```python
from build123d import *

# Parameters (mm, degrees)
SKETCH1_R           = 25.4
BOSS_EXTRUDE1_DEPTH = 584.2
SKETCH2_OUTSIDE_W   = 170.52
SKETCH2_OUTSIDE_H   = 170.52
SKETCH2_OUTSIDE_R   = 6.361935525
CUT_EXTRUDE1_DEPTH  = 50.8
SKETCH5_OUTSIDE_W   = 170.52
SKETCH5_OUTSIDE_H   = 170.52
SKETCH5_OUTSIDE_R   = 6.377907631
CUT_EXTRUDE4_DEPTH  = 50.8


with BuildPart() as part:
    # Sketch1 → Boss-Extrude1 (new body)
    with BuildSketch(Plane.XY):
        Circle(SKETCH1_R)
    extrude(amount=BOSS_EXTRUDE1_DEPTH)

    # Sketch2 outside → Cut-Extrude1 (cut)
    with BuildSketch(Plane.XY):
        Rectangle(SKETCH2_OUTSIDE_W, SKETCH2_OUTSIDE_H)
        Circle(SKETCH2_OUTSIDE_R, mode=Mode.SUBTRACT)
    extrude(amount=CUT_EXTRUDE1_DEPTH, mode=Mode.SUBTRACT)

    # Sketch5 outside → Cut-Extrude4 (cut)
    with BuildSketch(Plane.XY.offset(584.2)):
        Rectangle(SKETCH5_OUTSIDE_W, SKETCH5_OUTSIDE_H)
        Circle(SKETCH5_OUTSIDE_R, mode=Mode.SUBTRACT)
    extrude(amount=-CUT_EXTRUDE4_DEPTH, mode=Mode.SUBTRACT)


solid = part.part
```
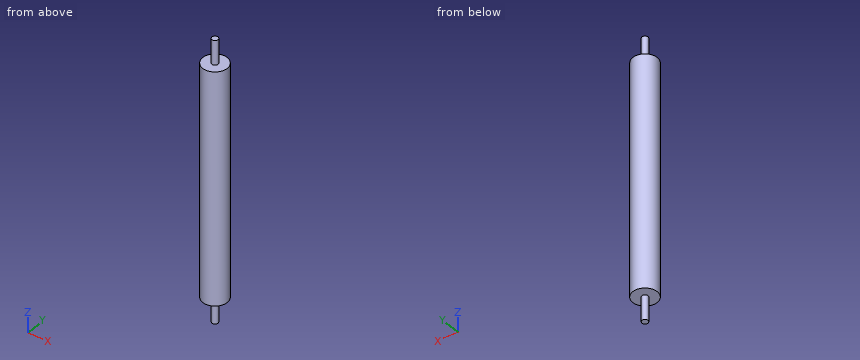
Part model, mm, in its own coordinate system. Round coordinates to 2 decimals unless told otherwise and drop trailing zeros. Order: outer loops, then holes, each group sorted by start corner. A loop starts at its lowest first (then second) coordinate and runs counter-clockwise, first axis right, second up. Notation, with made-up numbers: M -5.5,5.25 L -0.5,5.25 A8 ccw -0.5,17.25 Z; hole C 19,-1 d8. An arc over 180 degrees is marked long. Answer in a Markdown table with one row per item. Add a question column.
Q1. Cut at D-D on z = 539.5. Give the cut face in (x, y), and give its area (3 significant figures).
Q2. Pin check, flat tips, straight feed: pin 1 (10 mm diameter, centred on x = -3, y = -17, fed in from -Z); pin 2 (12 mm diameter, centred on x = 8, y = 11.5, fed in from +Z); pin 3 (10 mm diameter, centred on x = -14.5, z = 146, fed in from +Y). Stop position of each tip, or through.
Q3. Cut at A-A on y = 0. Give the cut face in (x, z), and give its area (3 significant figures).
Q4. Cut at C-C on z = 56.5. Give the cut face in (x, y).
Q5. Wall check: L1, parallel to Z at x = -12.5, y = -2; L2, parallel to X at y = 15, z = 90.5; L3, parallel to Y at x = 0.5, z = 231.5. Give the ranges that are in metal, low to high. Write a range as from..to.
Established:
| question | item | result |
|---|---|---|
| 1 | outline | C 0,0 d12.76 |
| 1 | area | 128 mm2 |
| 2 | pin 1 | stops at z = 50.8 |
| 2 | pin 2 | stops at z = 533.4 |
| 2 | pin 3 | stops at y = 23.56 |
| 3 | outline | M -25.4,50.8 L -6.36,50.8 L -6.36,0 L 6.36,0 L 6.36,50.8 L 25.4,50.8 L 25.4,533.4 L 6.38,533.4 L 6.38,584.2 L -6.38,584.2 L -6.38,533.4 L -25.4,533.4 Z |
| 3 | area | 25,800 mm2 |
| 4 | outline | C 0,0 d50.8 |
| 5 | L1 | z = 50.8..533.4 |
| 5 | L2 | x = -20.5..20.5 |
| 5 | L3 | y = -25.4..25.4 |
